Build history of the part. All positions in model axes, mm. A direction names the side the tool comes from. Give positions to 0.01 mm unless a question says otherwise; leave off trailing zeros. Order: outer loops, then holes, each group sorted by start corner. A loop starts at its lowest first (then second) coordinate and runs counter-clockwise, first axis right, second up. Notation, with made-up numbers: (31.25, 60.5) - (87.25, 60.5) arc R12 cw to (87.25, 68.5) - close; hole circle Ø6 at (-13.75, 77.5). An arc over 180 degrees is marked (long way). Use a Markdown table: item, result.
from build123d import *

# Parameters (mm, degrees)
BOSS_EXTRUDE2_DEPTH = 2.1082
BOSS_EXTRUDE3_DEPTH = 0.9
SKETCH13_W          = 5.200208993
SKETCH13_H          = 1.5
BOSS_EXTRUDE4_DEPTH = 6.35
SKETCH16_W          = 2.54
SKETCH16_H          = 1.5
BOSS_EXTRUDE5_DEPTH = 5.45


with BuildPart() as part:
    # Sketch6 → Boss-Extrude2 (new body)
    with BuildSketch(Plane(origin=(0, 0, 0), x_dir=(1, 0, 0), z_dir=(0, 1, 0))):
        with BuildLine():
            Line((3.1496, 3.175), (3.1496, 8.27377964))
            Line((3.1496, 8.27377964), (-5.741348421, 8.27377964))
            Line((-5.741348421, 8.27377964), (-8.59506403, 5.42006403))
            ThreePointArc((-8.59506403, 5.42006403), (-9.283317516, 4.390019898), (-9.525, 3.175))
            Line((-9.525, 3.175), (-9.525, -1.92377964))
            Line((-9.525, -1.92377964), (-6.989909723, -1.92377964))
            Line((-6.989909723, -1.92377964), (3.1496, -1.92377964))
            Line((3.1496, -1.92377964), (3.1496, 3.175))
        make_face()
    extrude(amount=BOSS_EXTRUDE2_DEPTH)

    # Sketch7 → Boss-Extrude3 (add)
    with BuildSketch(Plane.XZ):
        with BuildLine():
            Line((-2.050608993, 1.92377964), (-2.050608993, 0.42377964))
            ThreePointArc((-2.050608993, 0.42377964), (-0.881374643, -4.411978027), (-4.017957094, -8.27377964))
            Line((-4.017957094, -8.27377964), (6.35, -8.27377964))
            ThreePointArc((6.35, -8.27377964), (11.44877964, -3.175), (6.35, 1.92377964))
            Line((6.35, 1.92377964), (-2.050608993, 1.92377964))
        make_face()
    extrude(amount=BOSS_EXTRUDE3_DEPTH)

    # Sketch10 → Revolve2 (revolve)
    with BuildSketch(Plane.XY.offset(-3.175), mode=Mode.PRIVATE) as revolve2_sk:
        with BuildLine():
            Line((-6.35, 0), (-6.35, -1.065979307))
            ThreePointArc((-6.35, -1.065979307), (-5.088839039, -0.786386653), (-4.064, 0))
            Line((-4.064, 0), (-6.35, 0))
        make_face()
    revolve(revolve2_sk.sketch.rotate(Axis((-6.35, 0, -3.175), (0, -1, 0)), 180), axis=Axis((-6.35, 0, -3.175), (0, -1, 0)))

    # Sketch11 → Revolve4 (revolve)
    with BuildSketch(Plane.XY.offset(-3.175), mode=Mode.PRIVATE) as revolve4_sk:
        with BuildLine():
            Line((6.35, -0.9), (6.35, -2.083581452))
            ThreePointArc((6.35, -2.083581452), (7.929346537, -1.776499661), (9.278562256, -0.9))
            Line((9.278562256, -0.9), (6.35, -0.9))
        make_face()
    revolve(revolve4_sk.sketch.rotate(Axis((6.35, -0.9, -3.175), (0, -1, 0)), 180), axis=Axis((6.35, -0.9, -3.175), (0, -1, 0)))

    # Sketch12 → Cut-Revolve1 (revolve, cut)
    with BuildSketch(Plane.XY.offset(-3.175), mode=Mode.PRIVATE) as cut_revolve1_sk:
        with BuildLine():
            Line((8.89, 0), (6.35, 0))
            Line((6.35, 0), (6.35, -1.184421452))
            ThreePointArc((6.35, -1.184421452), (7.751289957, -0.873762947), (8.89, 0))
        make_face()
    revolve(cut_revolve1_sk.sketch.rotate(Axis((6.35, 0, -3.175), (0, -1, 0)), 180), axis=Axis((6.35, 0, -3.175), (0, -1, 0)), mode=Mode.SUBTRACT)

    # Sketch13 → Boss-Extrude4 (add)
    with BuildSketch(Plane.XZ):
        with Locations((0.549495504, 1.17377964)):
            Rectangle(SKETCH13_W, SKETCH13_H)
    extrude(amount=BOSS_EXTRUDE4_DEPTH)

    # Sketch16 → Boss-Extrude5 (add)
    with BuildSketch(Plane.XZ.offset(0.9)):
        with Locations((0, -7.52377964)):
            Rectangle(SKETCH16_W, SKETCH16_H)
    extrude(amount=BOSS_EXTRUDE5_DEPTH)

    # Mirror1: part across plane


with BuildPart() as part_1:
    add(part.part)
    add(part.part.mirror(Plane(origin=(3.1496, -6.35, 1.92377964), x_dir=(0, 0, 1), z_dir=(0, 1, 0))))


solid = part_1.part
1) Slice it at D-D (y = -12.25). State how many separate pieces and enclosed holes the cut face has, and give its area (3 significant figures).
Computed:
| item | result |
|---|---|
| separate pieces | 2 |
| enclosed holes | 1 |
| area | 118 mm² |
2) Two-plate mould, pull along X, no slides. Class faces 5 (the flat face through (-7.148, -13.739, -6.867)), 6 (the cylindrical face through (-0.866, -0.444, -4.341)), 7 (the flat face through (0, -6, -6.774)): +X half, -X half, draft (parallel to the pull), parting line (faces both ways), or undercut.
Computed:
| item | result |
|---|---|
| face 5 | -X half |
| face 6 | undercut |
| face 7 | draft |
3) Wall check: line 1 (Y direction, x = 1.25, z = -6.25); line 2 (Y direction, x = 4, z = 1.5); line 3 (X direction, y = -13.25, z = 1) (3 decimals). Give the ranges that are in metal, low to high. Write a range as from..to.
Computed:
| item | result |
|---|---|
| line 1 | y = -14.81..-11.8, -0.9..2.11 |
| line 2 | y = -12.7..-11.8, -0.9..0 |
| line 3 | x = -9.525..3.15 |
4) Tool access for faces 1 (the flat face through (3.15, -14, -3)), 2 (the flat face through (-4, 0, -2)), 3 (the flat face through (1, -6, 0.424)), 4 (the flat face through (-1.27, -6, -8)): list every direction of +Z, -Z, +X, -X, +Y, -Y with a clear straight run to the whole face (end or side of a thin tool).
Computed:
| item | result |
|---|---|
| face 1 | +Z, -Z, +X, -Y |
| face 2 | none |
| face 3 | +X, -X |
| face 4 | -Z, -X |
5) Slice it at A-A (x = 0.5). Write the cut outline in (y, z), and give its area (3 significant figures).
Computed:
| item | result |
|---|---|
| outline | (-14.81, -8.27) - (2.11, -8.27) - (2.11, 1.92) - (-14.81, 1.92) - close; hole (-11.8, -6.77) - (-0.9, -6.77) - (-0.9, 0.42) - (-11.8, 0.42) - close |
| area | 94.1 mm² |
6) Slice it at C-C (x = -3). Write the cut outline in (y, z).
Computed:
| item | result |
|---|---|
| outline | (-14.81, -8.27) - (-11.8, -8.27) - (-11.8, -7.67) - (-12.7, -7.67) - (-12.7, 1.92) - (-14.81, 1.92) - close; (-0.9, -8.27) - (2.11, -8.27) - (2.11, 1.92) - (0, 1.92) - (0, -7.67) - (-0.9, -7.67) - close |
7) Pin check, flat tips, straight feed: P1, Ø0.5, axis at y = -5.5, z = -8, coming from the -X side; P2, Ø2, axis at x = -4.5, y = -5.5, coming from the -Z side; P3, Ø1.1, axis at y = 1, z = -1.5, coming from the +X side; P4, Ø3, axis at x = 6, z = -5.5, coming from the +Y side. Stop position of each tip, or through.
Computed:
| item | result |
|---|---|
| P1 | stops at x = -1.27 |
| P2 | passes through |
| P3 | stops at x = 3.15 |
| P4 | stops at y = 0 |
8) Slice it at B-B (y = -3.75). Write the cut outline in (x, z), and give its area (3 significant figures).
Computed:
| item | result |
|---|---|
| outline | (-2.05, 0.42) - (3.15, 0.42) - (3.15, 1.92) - (-2.05, 1.92) - close; (-1.27, -8.27) - (1.27, -8.27) - (1.27, -6.77) - (-1.27, -6.77) - close |
| area | 11.6 mm² |
